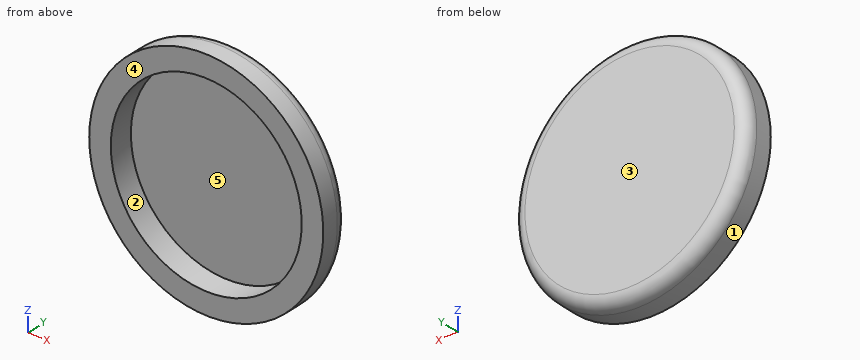
Autodesk Inventor part; units mm, degrees
ref_plane "YZ Plane" through (0, 0, 0) normal (1, 0, 0) x (0, 1, 0)
ref_plane "XZ Plane" through (0, 0, 0) normal (0, 1, 0) x (-1, 0, 0)
ref_plane "XY Plane" through (0, 0, 0) normal (0, 0, 1) x (1, 0, 0)
sketch "Эскиз1" plane through (0, 0, 0) normal (0, 1, 0) x (-1, 0, 0)
  circle A0 centre (0, 0) radius 9.5
  circle A1 centre (0, 0) radius 7.75
  dimension "d0" = 19
  dimension "d1" = 15.5
extrude "Выдавливание1" add sketch "Эскиз1" along normal blind 2
sketch "Эскиз2" plane through (0, 2, 0) normal (0, 1, 0) x (1, 0, 0)
  circle A0 centre (0, 0) radius 9.5
extrude "Выдавливание2" add sketch "Эскиз2" along normal blind 0.4
fillet "Сопряжение1" radius 1 1 edges at (-9.5, 2.4, 0)
properties part number "derz magnit"
Here's how the part is built. I have some questions about the finished solid (model axes, mm). Face numbers are marked on the shaded views. A direction names the side the tool comes from. Give positions to 0.01 mm unless a question says otherwise; leave off trailing zeros. Order: outer loops, then holes, each group sorted by start corner. A loop starts at its lowest first (then second) coordinate and runs counter-clockwise, first axis right, second up. Notation, with made-up numbers: M -16,0.25 L 1,0.25 A28 cw 1,18.25 Z; hole C 67,-35.5 d10. An arc over 180 degrees is marked long. Use a Markdown table: item, result. Add a question column.
1. I need wall thicknesses on probe 1 along Z at (x, y) = (0, 1.05); probe 2 along Y at (x, z) = (4.75, -1.25); probe 3 along X at (y, z) = (0.45, -3.5). Which ranges of each line are inside material? Lowest first, please. Write a range as from..to.
2. Suppose I cut it at A-A (z = 0). List the corners of the cut face in (x, y) for me, and give its area (3 significant figures).
3. If we mould it in two halves opening along Z, with no side actions, what happens to the marked faces 1, 2 and 3? For each: +Z half, -Z half, draft (parallel to the pull), parting line (faces both ways), or undercut.
4. Suppose I cut it at B-B (x = 0). List the corners of the cut face in (y, z) for me.
5. Suppose I cut it at C-C (y = 0.9). List the corners of the cut face in (x, z) for me, and give its area (3 significant figures).
6. On a 3-axis mill with a long thin cutter (end or side, diameter ignored), from which of +Z, -Z, +X, -X, +Y, -Y can I reach the whole of each face in a straight line? I mean the marked faces 4 and 5. Say none if no direction works.
7. For pin 1 Ø1 at (x, y) = (-4.5, 2) entering from +Z, with a flat end and sliding along its axis, tell me the tip position at first contact or that it passes through.
Results list:
| question | item | result |
|---|---|---|
| 1 | probe 1 | z = -9.5..-7.75, 7.75..9.5 |
| 1 | probe 2 | y = 2..2.4 |
| 1 | probe 3 | x = -8.83..-6.91, 6.91..8.83 |
| 2 | outline | M -9.5,0 L -7.75,0 L -7.75,2 L 7.75,2 L 7.75,0 L 9.5,0 L 9.5,1.4 A1 ccw 8.5,2.4 L -8.5,2.4 A1 ccw -9.5,1.4 Z |
| 2 | area | 14.2 mm² |
| 3 | face 1 | parting line |
| 3 | face 2 | undercut |
| 3 | face 3 | draft |
| 4 | outline | M 0,-9.5 L 1.4,-9.5 A1 ccw 2.4,-8.5 L 2.4,8.5 A1 ccw 1.4,9.5 L 0,9.5 L 0,7.75 L 2,7.75 L 2,-7.75 L 0,-7.75 Z |
| 5 | outline | C 0,0 d19; hole C 0,0 d15.5 |
| 5 | area | 94.8 mm² |
| 6 | face 4 | +Z, -Z, +X, -X, -Y |
| 6 | face 5 | -Y |
| 7 | pin 1 | stops at z = 8.52 |
